Answer from the drawing. Dimensions are ordinates in mm from the lowest x, y and z of the part. A direction names the side the tool comes from. Round coordinates to 2 decimals unless told otherwise and drop trailing zeros. Order: outer loops, then holes, each group sorted by start corner. A loop starts at its lowest first (then second) coordinate and runs counter-clockwise, first axis right, second up. Notation, with made-up numbers: (47, -32.5) - (87, -32.5) arc R24 ccw to (87, -19.5) - close; hole circle Ø5 at (-33.5, 23). An arc over 180 degrees is marked (long way). One line per question, with ' | ' between items. Start each with the question number.
1) The part is cut by section D-D, the plane x = 491.5. Give the vertices of the cut face in (y, z).
2) Straight lines are drawn through the part: line 1 (Y direction, x = 142, z = 111); line 2 (Z direction, x = 464.5, y = 78); line 3 (X direction, y = 80, z = 99). For each, find the intervals that lie inside material, in ascending order. Write a range as from..to.
3) The part is cut by section B-B, the plane z = 89. Give the vertices of the cut face in (x, y), plus the area to 3 significant figures.
4) For the marked faces 1 and 2, determine the directions among +Z, -Z, +X, -X, +Y, -Y from which every point of the face is accessible in a straight line to the end or side of a thin tool.
5) The part is cut by section A-A, the plane x = 429.5. Give the vertices of the cut face in (y, z), plus the area to 3 significant figures.
6) Flat-ended cylindrical pins translate along their axes: pin 1 (14.5 mm diameter, centred on y = 113, z = 106.5, fed in from -X); pin 2 (2 mm diameter, centred on x = 271.5, y = 65, fed in from -Z). Find the tip coordinate at first contact, or state that the pin passes through.
7) The part is cut by section C-C, the plane y = 27.5. Give the vertices of the cut face in (x, z).
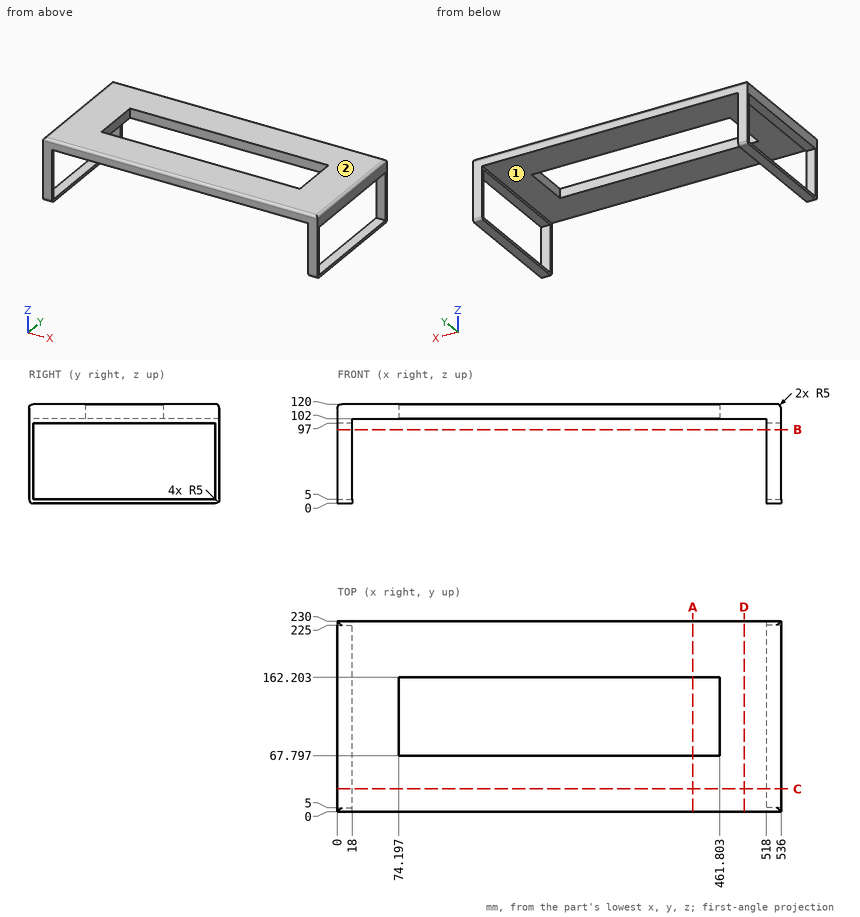
Values:
1) outline: (0, 102) - (230, 102) - (230, 115) arc R5 ccw to (225, 120) - (5, 120) arc R5 ccw to (0, 115) - close
2) line 1: y = 0..67.8, 162.2..230 | line 2: z = 102..120 | line 3: x = 0..18, 518..536
3) outline: (0, 0) - (18, 0) - (18, 5) - (0, 5) - close; (0, 225) - (18, 225) - (18, 230) - (0, 230) - close; (518, 0) - (536, 0) - (536, 5) - (518, 5) - close; (518, 225) - (536, 225) - (536, 230) - (518, 230) - close | area: 360 mm^2
4) face 1: -Z, +Y, -Y | face 2: +Z, +X, -X, +Y, -Y
5) outline: (0, 102) - (67.8, 102) - (67.8, 120) - (5, 120) arc R5 ccw to (0, 115) - close; (162.2, 102) - (230, 102) - (230, 115) arc R5 ccw to (225, 120) - (162.2, 120) - close | area: 2,430 mm^2
6) pin 1: stops at x = 0 | pin 2: stops at z = 102
7) outline: (0, 0) - (18, 0) - (18, 5) - (0, 5) - close; (0, 97) - (18, 97) - (18, 102) - (518, 102) - (518, 97) - (536, 97) - (536, 115) arc R5 ccw to (531, 120) - (5, 120) arc R5 ccw to (0, 115) - close; (518, 0) - (536, 0) - (536, 5) - (518, 5) - close
